Autodesk Inventor part; units mm, degrees
ref_plane "YZ Plane" through (0, 0, 0) normal (1, 0, 0) x (0, 1, 0)
ref_plane "XZ Plane" through (0, 0, 0) normal (0, 1, 0) x (-1, 0, 0)
ref_plane "XY Plane" through (0, 0, 0) normal (0, 0, 1) x (1, 0, 0)
sketch "Sketch1" plane through (0, 0, 0) normal (0, 1, 0) x (-1, 0, 0)
  line L0 (-177.8, 330.2) -> (177.8, 330.2)
  line L1 (177.8, 330.2) -> (177.8, -330.2)
  line L2 (177.8, -330.2) -> (-177.8, -330.2)
  line L3 (-177.8, -330.2) -> (-177.8, 330.2)
  line L4 (-177.8, 330.2) -> (177.8, -330.2) construction
  line L5 (177.8, 330.2) -> (-177.8, -330.2) construction
  point P0 (0, 0)
  dimension "d0" = 355.6
  dimension "d1" = 660.4
extrude "Extrusion1" add sketch "Sketch1" along normal blind 114.3 and the other way blind 25.4
sketch "Sketch2" plane through (177.8, -25.4, -330.2) normal (1, 0, 0) x (0, 0, -1)
  line L0 (-584.2, 25.4) -> (-76.2, 25.4) construction
  line L1 (-584.2, -50.8) -> (-76.2, -50.8)
  line L2 (-76.2, 101.6) -> (-584.2, 101.6)
  arc A0 (-584.2, 101.6) -> (-584.2, -50.8) centre (-584.2, 25.4) ccw
  arc A1 (-76.2, -50.8) -> (-76.2, 101.6) centre (-76.2, 25.4) ccw
  line L3 (-330.2, 25.4) -> (177.8, 25.4) construction
  line L4 (-330.2, 25.4) -> (-330.2, 0) construction
  line L5 (-660.4, 0) -> (0, 0) construction
  point P0 (-330.2, 25.4)
  dimension "d6" = 254
  dimension "d7" = 0
  dimension "d8" = 152.4
  dimension "d9" = 25.4
extrude "Extrusion2" add sketch "Sketch2" along normal blind 101.6
sketch "Sketch3" plane through (279.4, -25.4, -330.2) normal (1, 0, 0) x (0, 0, -1)
  circle A0 centre (-584.2, 25.4) radius 63.5
  circle A1 centre (-76.2, 25.4) radius 63.5
  arc A2 (-584.2, 101.6) -> (-584.2, -50.8) centre (-584.2, 25.4) ccw construction
  arc A3 (-76.2, -50.8) -> (-76.2, 101.6) centre (-76.2, 25.4) ccw construction
  point P0 (-330.2, 25.4)
  dimension "d12" = 127
extrude "Extrusion3" add sketch "Sketch3" along normal blind 6.35
sketch "Sketch4" plane through (285.75, 0, 254) normal (1, 0, 0) x (0, 0, -1)
  line L0 (0, 0) -> (-215.5261, 215.5261) construction
  line L1 (46.7237, 60.1941) -> (-192.1643, 245.6232)
  line L2 (-245.6232, 192.1643) -> (-60.1941, -46.7237)
  arc A0 (-60.1941, -46.7237) -> (46.7237, 60.1941) centre (0, 0) ccw
  arc A1 (-192.1643, 245.6232) -> (-245.6232, 192.1643) centre (-215.5261, 215.5261) ccw
  arc A2 (0, 76.2) -> (0, -76.2) centre (0, 0) ccw construction
  line L3 (0, 0) -> (-144.2559, 0) construction
  line L4 (508, 0) -> (508, 304.8) construction
  line L5 (583.6023, 9.525) -> (545.8012, 309.5625)
  line L6 (470.1988, 309.5625) -> (432.3977, 9.525)
  arc A3 (432.3977, 9.525) -> (583.6023, 9.525) centre (508, 0) ccw
  arc A4 (545.8012, 309.5625) -> (470.1988, 309.5625) centre (508, 304.8) ccw
  circle A5 centre (508, 0) radius 63.5 construction
  point P0 (254, 0)
  point P1 (-107.7631, 107.7631)
  point P2 (508, 152.4)
  dimension "d15" = 304.8
  dimension "d17" = 38.1
  dimension "d20" = 45
extrude "Extrusion4" add sketch "Sketch4" along normal blind 50.8
mirror "Mirror1" about plane through (0, 0, 0) normal (1, 0, 0) of "Extrusion2", "Extrusion4", "Extrusion3"
properties part number "Dimensions(Roughly)" material "Air"
Geometry check sheet. Reference: the model listing, model coordinates, mm. A direction names the side the tool comes from. Round coordinates to 2 decimals unless told otherwise and drop trailing zeros. Order: outer loops, then holes, each group sorted by start corner. A loop starts at its lowest first (then second) coordinate and runs counter-clockwise, first axis right, second up. Notation, with made-up numbers: M 61,80 L 71,80 A25 cw 71,98 Z; hole C -30,-14.75 d10. An arc over 180 degrees is marked long. Answer in a Markdown table with one row per item. Add a question column.
Item 1: Sectioned sample at D-D, the plane x = 86. Enter the section's corners in (y, z), plus the area to 3 significant figures.
Item 2: Draft check along Z on faces 1 (the face through (310.79, -76.18, -255.81)), 2 (the face through (-227.89, 1.68, 330.18)), 3 (the face through (2, 114.3, 5)). Enter one of: released by +Z, released by -Z, zero draft, split by the parting line, or undercut.
Item 3: Depth check by flat-ended pin: pin 1 Ø3 at (x, y) = (50.5, 45) entering from +Z; pin 2 Ø2 at (x, z) = (43.5, 96.5) entering from -Y; pin 3 Ø12 at (y, z) = (-18, 93.5) entering from +X. Enter the tip coordinate at first touch or a pass-through.
Item 4: Sectioned sample at B-B, the plane z = 368. Enter the section's corners in (x, y), plus the area to 3 significant figures.
Item 5: Sectioned sample at A-A, the plane y = 97.5. Enter the section's corners in (x, z).
Item 6: Sectioned sample at C-C, the plane z = -238.5. Enter the section's corners in (x, y), plus the area to 3 significant figures.
Item 7: Material ranges on L1, parallel to X at y = 32.5, z = 316.5; L2, parallel to X at y = -33, z = 131.5; L3, parallel to X at y = 111.5, z = 365, recorded low to high. Write a range as [from, to].
Item 8: Set-up check for faces 4 (the face through (310.794, 157.443, -310.966)), 5 (the face through (282.53, 24.32, -312.66)), 6 (the face through (310.794, 161.644, -197.563)): record each of +Z, -Z, +X, -X, +Y, -Y from which the full face is reachable in a straight line by a thin tool's end or side.
Filled in:
| question | item | result |
|---|---|---|
| 1 | outline | M -25.4,-330.2 L 114.3,-330.2 L 114.3,330.2 L -25.4,330.2 Z |
| 1 | area | 92,300 mm² |
| 2 | face 1 | undercut |
| 2 | face 2 | released by +Z |
| 2 | face 3 | zero draft |
| 3 | pin 1 | stops at z = 330.2 |
| 3 | pin 2 | stops at y = -25.4 |
| 3 | pin 3 | stops at x = 279.4 |
| 4 | outline | M -336.55,22.59 L -285.75,22.59 L -285.75,184.95 L -336.55,184.95 Z; M 285.75,22.59 L 336.55,22.59 L 336.55,184.95 L 285.75,184.95 Z |
| 4 | area | 16,500 mm² |
| 5 | outline | M -336.55,-318.52 L -285.75,-318.52 L -285.75,-189.48 L -336.55,-189.48 Z; M -336.55,255.34 L -285.75,255.34 L -285.75,426.14 L -336.55,426.14 Z; M -177.8,-330.2 L 177.8,-330.2 L 177.8,330.2 L -177.8,330.2 Z; M 285.75,-318.52 L 336.55,-318.52 L 336.55,-189.48 L 285.75,-189.48 Z; M 285.75,255.34 L 336.55,255.34 L 336.55,426.14 L 285.75,426.14 Z |
| 6 | outline | M -336.55,-74.61 L -285.75,-74.61 L -285.75,-61.58 L -279.4,-61.58 L -279.4,-76.2 L -177.8,-76.2 L -177.8,-25.4 L 177.8,-25.4 L 177.8,-76.2 L 279.4,-76.2 L 279.4,-61.58 L 285.75,-61.58 L 285.75,-74.61 L 336.55,-74.61 L 336.55,339.6 L 285.75,339.6 L 285.75,61.58 L 279.4,61.58 L 279.4,76.2 L 177.8,76.2 L 177.8,114.3 L -177.8,114.3 L -177.8,76.2 L -279.4,76.2 L -279.4,61.58 L -285.75,61.58 L -285.75,339.6 L -336.55,339.6 Z |
| 6 | area | 124,000 mm² |
| 7 | L1 | x = [-336.55, -285.75], [-279.4, 279.4], [285.75, 336.55] |
| 7 | L2 | x = [-279.4, -177.8], [177.8, 279.4] |
| 7 | L3 | x = [-336.55, -285.75], [285.75, 336.55] |
| 8 | face 4 | -Z, +X, +Y |
| 8 | face 5 | none |
| 8 | face 6 | +X, +Y |
